Read the model definition and answer for the solid it produces. Units are mm, in the model's axes. Coordinates: 2 decimals unless noted, no trailing zeros. Write each loop counter-clockwise with the first axis right and the second up, starting at its lowest first coordinate (ties: lowest second). Pieces come first, ordered by that corner, then holes. Notation, with made-up numbers: (41.5, 77.5) - (83.5, 77.5) arc R26 ccw to (83.5, 116.5) - close; hole circle Ø8 at (32, 29.5). An arc over 180 degrees is marked (long way). Use a Markdown table: item, result.
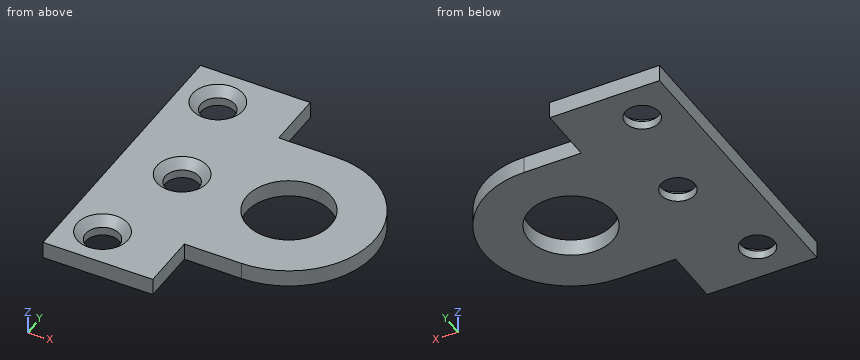
from build123d import *

# Parameters (mm, degrees)
SKETCH1_R           = 7.9375
SKETCH1_R_2         = 3.175
BOSS_EXTRUDE1_DEPTH = 3.175
CHAMFER1_SIZE       = 1.5875


with BuildPart() as part:
    # Sketch1 → Boss-Extrude1 (new body)
    with BuildSketch(Plane.XY):
        with BuildLine():
            Line((0, 16.1925), (-10.795, 16.1925))
            Line((-10.795, 16.1925), (-10.795, 26.9875))
            Line((-10.795, 26.9875), (-31.4325, 26.9875))
            Line((-31.4325, 26.9875), (-31.4325, -26.9875))
            Line((-31.4325, -26.9875), (-10.795, -26.9875))
            Line((-10.795, -26.9875), (-10.795, -16.1925))
            Line((-10.795, -16.1925), (0, -16.1925))
            ThreePointArc((0, -16.1925), (16.1925, 0), (0, 16.1925))
        make_face()
        Circle(SKETCH1_R, mode=Mode.SUBTRACT)
        with Locations((-24.209375, 19.764375)):
            Circle(SKETCH1_R_2, mode=Mode.SUBTRACT)
        with Locations((-20.081875, 0)):
            Circle(SKETCH1_R_2, mode=Mode.SUBTRACT)
        with Locations((-24.209375, -19.764375)):
            Circle(SKETCH1_R_2, mode=Mode.SUBTRACT)
    extrude(amount=BOSS_EXTRUDE1_DEPTH)

    # Chamfer1
    chamfer1_edges = [part.edges().sort_by_distance(p)[0] for p in [
        (-27.384375, 19.764375, 3.175),
        (-23.256875, 0, 3.175),
        (-27.384375, -19.764375, 3.175),
    ]]
    chamfer(chamfer1_edges, length=CHAMFER1_SIZE)


solid = part.part
(1) A cutting plane is placed at A-A, the plane y = 7. Write down the section's boundary in (x, z) (1 decimal), and give its area (3 significant figures).
Report:
| item | result |
|---|---|
| outline | (-31.4, 0) - (-3.7, 0) - (-3.7, 3.2) - (-31.4, 3.2) - close; (3.7, 0) - (14.6, 0) - (14.6, 3.2) - (3.7, 3.2) - close |
| area | 122 mm² |
(2) Each of these flat-tipped pins is pushed along its axis until it touches: P1, Ø6, axis at x = 4, y = -11.5, coming from the -Z side; P2, Ø1, axis at y = 18.5, z = 2, coming from the +X side (3 decimals); P3, Ø3, axis at x = -26, y = -19, coming from the +Z side; P4, Ø5, axis at x = -24.21, y = 19.76, coming from the +Z side. Where does it stop, or does it pass through?
Report:
| item | result |
|---|---|
| P1 | stops at z = 0 |
| P2 | stops at x = -10.795 |
| P3 | stops at z = 1.86 |
| P4 | passes through |
(3) A cutting plane is placed at B-B, the plane x = 7. Write down the section's boundary in (y, z) (3 decimals), and give its area (3 significant figures).
Report:
| item | result |
|---|---|
| outline | (-14.601, 0) - (-3.742, 0) - (-3.742, 3.175) - (-14.601, 3.175) - close; (3.742, 0) - (14.601, 0) - (14.601, 3.175) - (3.742, 3.175) - close |
| area | 69.0 mm² |
(4) A cutting plane is placed at C-C, the plane z = 0.6. Count the separate pieces of the cut face and the enclosed holes in it, and give its area (3 significant figures).
Report:
| item | result |
|---|---|
| separate pieces | 1 |
| enclosed holes | 4 |
| area | 1,580 mm² |
(5) Straight lines are drawn through the part: L1, parallel to X at y = 1, z = 2.65; L2, parallel to X at y = -0.5, z = 0.65; L3, parallel to Y at x = -23, z = 2.1. For each, find the intervals that lie inside material, in ascending order.
Report:
| item | result |
|---|---|
| L1 | x = -31.43 to -24.2, -15.96 to -7.87, 7.87 to 16.16 |
| L2 | x = -31.43 to -23.22, -16.95 to -7.92, 7.92 to 16.18 |
| L3 | y = -26.99 to -23.25, -16.28 to -2.25, 2.25 to 16.28, 23.25 to 26.99 |
